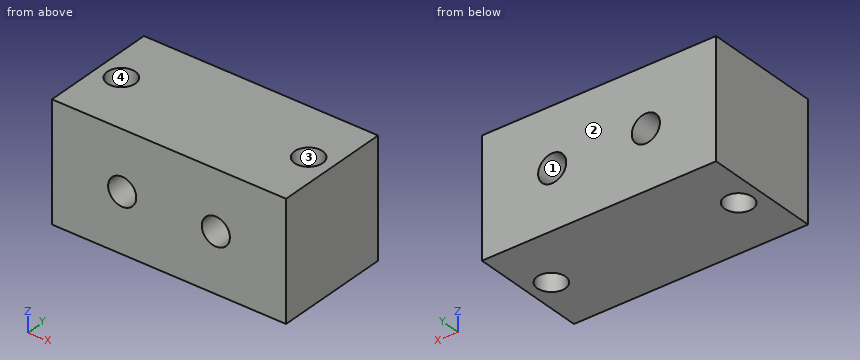
Autodesk Fusion 360 part; units mm, degrees
sketch "Sketch1" plane through (0, 0, 0) normal (1, 0, 0) x (0, 0, -1)
  line L0 (12.5, 12.5) -> (-12.5, 12.5)
  line L1 (-12.5, 12.5) -> (-12.5, -12.5)
  line L2 (-12.5, -12.5) -> (12.5, -12.5)
  line L3 (12.5, -12.5) -> (12.5, 12.5)
  line L4 (12.5, 12.5) -> (-12.5, -12.5) construction
  line L5 (-12.5, 12.5) -> (12.5, -12.5) construction
  dimension "d1" = 25
  dimension "d2" = 25
extrude "Extrude1" add sketch "Sketch1" along normal blind 50
sketch "Sketch2" plane through (0, 0, 12.5) normal (0, 0, 1) x (1, 0, 0)
  line L0 (0, 12.5) -> (0, -12.5)
  line L1 (0, -12.5) -> (50, -12.5)
  line L2 (50, -12.5) -> (50, 12.5)
  line L3 (50, 12.5) -> (0, 12.5)
  circle A0 centre (5, 0) radius 3
  line L4 (25, 12.5) -> (25, -12.5) construction
  circle A1 centre (45, 0) radius 3
  dimension "d5" = 6
  dimension "d8" = 20
sketch "Sketch3" plane through (0, 12.5, 0) normal (0, 1, 0) x (-1, 0, 0)
  line L0 (0, -12.5) -> (0, 12.5)
  line L1 (0, 12.5) -> (-50, 12.5)
  line L2 (-50, 12.5) -> (-50, -12.5)
  line L3 (-50, -12.5) -> (0, -12.5)
  line L4 (-25, -12.5) -> (-25, 12.5) construction
  circle A0 centre (-15, 0) radius 3
  circle A1 centre (-35, 0) radius 3
  dimension "d9" = 6
  dimension "d10" = 10
extrude "Extrude2" cut sketch "Sketch3" against normal through all contours A0 | A1
extrude "Extrude3" cut sketch "Sketch2" against normal through all contours A0 | A1
Build history of the part. All positions in model axes, mm. Face numbers are marked on the shaded views. Give positions to 0.01 mm unless a question says otherwise; leave off trailing zeros. Order: outer loops, then holes, each group sorted by start corner. A loop starts at its lowest first (then second) coordinate and runs counter-clockwise, first axis right, second up. Notation, with made-up numbers: M -1,75.25 L 27,75.25 A18 ccw 27,83.25 Z; hole C 86,-7.75 d5. An arc over 180 degrees is marked long. Use one line per item in the form item = value.
1) Saw through at A-A (y = 0). Give the cut face in (x, z).
Calculated:
outline = M 0,-12.5 L 2,-12.5 L 2,12.5 L 0,12.5 Z; M 8,-12.5 L 42,-12.5 L 42,12.5 L 8,12.5 Z; M 48,-12.5 L 50,-12.5 L 50,12.5 L 48,12.5 Z; hole C 15,0 d6; hole C 35,0 d6
2) Saw through at B-B (x = 45). Give the cut face in (y, z), plus the area to 3 significant figures.
Calculated:
outline = M -12.5,-12.5 L -3,-12.5 L -3,12.5 L -12.5,12.5 Z; M 3,-12.5 L 12.5,-12.5 L 12.5,12.5 L 3,12.5 Z
area = 475 mm2
3) Two-plate mould, pull along Y, no slides. Class the marked faces 1, 2, 3 and 4: released by +Y, released by -Y, zero draft, split by the parting line, or undercut.
Calculated:
face_1 = zero draft
face_2 = released by +Y
face_3 = undercut
face_4 = undercut
4) Saw through at D-D (y = -4.5). Give the cut face in (x, z), plus the area to 3 significant figures.
Calculated:
outline = M 0,-12.5 L 50,-12.5 L 50,12.5 L 0,12.5 Z; hole C 15,0 d6; hole C 35,0 d6
area = 1,190 mm2
5) Probe probe 1 along X at (y, z) = (9.75, -1); probe 2 along Z at (x, y) = (35, -6.5). List the from-to ranges inside material, lowest first.
Calculated:
probe_1 = 0 to 12.17, 17.83 to 32.17, 37.83 to 50
probe_2 = -12.5 to -3, 3 to 12.5
6) Saw through at C-C (z = -6.75). Give the cut face in (x, y), plus the area to 3 significant figures.
Calculated:
outline = M 0,-12.5 L 50,-12.5 L 50,12.5 L 0,12.5 Z; hole C 5,0 d6; hole C 45,0 d6
area = 1,190 mm2
7) Drop a flat-ended pin along its axis: pin 1 (5 mm diameter, centred on x = 5, y = 0, fed in from +Z). Give the stop position or say it passes through.
Calculated:
pin_1 = through
